Can you work these out from the model? Positions are in its coordinate system, mm. Face numbers are marked on the shaded views. Coordinates: 2 decimals unless noted, no trailing zeros. Order: outer loops, then holes, each group sorted by start corner. A loop starts at its lowest first (then second) coordinate and runs counter-clockwise, first axis right, second up. Notation, with made-up numbers: (6, 30.25) -> (33, 30.25) arc R6 cw to (33, 36.25) -> close; hole circle Ø7 at (69.5, 33.25). An arc over 180 degrees is marked (long way). Return JSON: item names as keys, results as strings. Group by question number.
1) If we section it at D-D, the plane z = -32.5: Please give me the cut outline in (x, y).
2) If we section it at C-C, the plane y = 14: Please give me the cut outline in (x, z).
3) If we section it at B-B, the plane z = 8.5: Please give me the cut outline in (x, y).
4) Thinking about a two-plate mould opening in Z: for the marked faces 1, 2, 3 and 4, which applies, +Z half, -Z half, draft (parallel to the pull), parting line (faces both ways), or undercut?
5) If I drill on probe 1 along Z at (x, y) = (-8, 22); probe 2 along Y at (x, z) = (-40, -23); probe 3 along Z at (x, y) = (-13, 5.5), over which ranges is the centre line in solid material (lowest first)? Write a range as from..to.
6) If we section it at A-A, the plane x = -12: Please give me the cut outline in (y, z), then the cut area to 3 significant figures.
7) For pin 1 (8 mm diameter, centred on x = 1, y = 12, fed in from -Z); pin 2 (21 mm diameter, centred on y = 22, z = -0.5, fed in from +X); pin 3 (6 mm diameter, centred on x = 29, z = -23, fed in from +Y), each with a flat end and sliding along its axis, tell me the tip position at first contact or that it passes through.
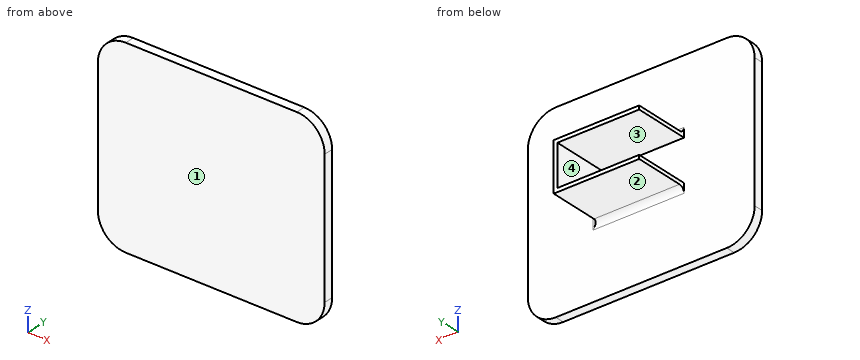
from build123d import *

# Parameters (mm, degrees)
SKETCH1_W           = 122
SKETCH1_H           = 102
BOSS_EXTRUDE1_DEPTH = 5
SKETCH2_W           = 46
SKETCH2_H           = 26
SKETCH2_W_2         = 42
SKETCH2_H_2         = 22
BOSS_EXTRUDE2_DEPTH = 30
SKETCH3_W           = 22
SKETCH3_H           = 30
CUT_EXTRUDE1_DEPTH  = 2
FILLET1_R           = 3
FILLET2_R           = 15


with BuildPart() as part:
    # Sketch1 → Boss-Extrude1 (new body)
    with BuildSketch(Plane(origin=(0, 0, 0), x_dir=(1, 0, 0), z_dir=(0, 1, 0))):
        Rectangle(SKETCH1_W, SKETCH1_H)
    extrude(amount=BOSS_EXTRUDE1_DEPTH)

    # Sketch2 → Boss-Extrude2 (add)
    with BuildSketch(Plane(origin=(0, 5, 0), x_dir=(1, 0, 0), z_dir=(0, 1, 0))):
        Rectangle(SKETCH2_W, SKETCH2_H)
        Rectangle(SKETCH2_W_2, SKETCH2_H_2, mode=Mode.SUBTRACT)
    extrude(amount=BOSS_EXTRUDE2_DEPTH)

    # Sketch3 → Cut-Extrude1 (cut)
    with BuildSketch(Plane.ZY.offset(23)):
        with Locations((0, 20)):
            Rectangle(SKETCH3_W, SKETCH3_H)
    extrude(amount=-CUT_EXTRUDE1_DEPTH, mode=Mode.SUBTRACT)

    # Fillet1
    fillet1_edges = [part.edges().sort_by_distance(p)[0] for p in [
        (0, 5, 13),
        (23, 5, 0),
        (0, 5, -13),
    ]]
    fillet(fillet1_edges, radius=FILLET1_R)

    # Fillet2
    fillet2_edges = [part.edges().sort_by_distance(p)[0] for p in [
        (-61, 2.5, -51),
        (61, 2.5, -51),
        (61, 2.5, 51),
        (-61, 2.5, 51),
    ]]
    fillet(fillet2_edges, radius=FILLET2_R)


solid = part.part
Result sheet:
{
 "1": {"outline": "(-61, 0) -> (61, 0) -> (61, 5) -> (-61, 5) -> close"},
 "2": {"outline": "(-23, -13) -> (23, -13) -> (23, 13) -> (-23, 13) -> (-23, 11) -> (21, 11) -> (21, -11) -> (-23, -11) -> close"},
 "3": {"outline": "(-61, 0) -> (61, 0) -> (61, 5) -> (26, 5) arc R3 cw to (23, 8) -> (23, 35) -> (21, 35) -> (21, 5) -> (-61, 5) -> close"},
 "4": {"face 1": "draft", "face 2": "-Z half", "face 3": "undercut", "face 4": "undercut"},
 "5": {"probe 1": "z = -13..-11, 11..13", "probe 2": "y = 0..5", "probe 3": "z = -14.34..-11, 11..14.34"},
 "6": {"outline": "(0, -51) -> (5, -51) -> (5, -16) arc R3 cw to (8, -13) -> (35, -13) -> (35, -11) -> (5, -11) -> (5, 11) -> (35, 11) -> (35, 13) -> (8, 13) arc R3 cw to (5, 16) -> (5, 51) -> (0, 51) -> close", "area": "634 mm2"},
 "7": {"pin 1": "stops at z = -13", "pin 2": "stops at x = 23", "pin 3": "stops at y = 5"}
}
